from build123d import *

# Parameters (mm, degrees)
F0_R     = 2
F1_DEPTH = 1
F2_R     = 15
F3_DEPTH = 99


with BuildPart() as f1:
    # F0 (on Top) → F1 (new body)
    with BuildSketch(Plane.XY):
        with BuildLine():
            ThreePointArc((-30, -29), (-29.707107, -29.707107), (-29, -30))
            Line((-29, -30), (29, -30))
            ThreePointArc((29, -30), (29.707107, -29.707107), (30, -29))
            Line((30, -29), (30, 29))
            ThreePointArc((30, 29), (29.707107, 29.707107), (29, 30))
            Line((29, 30), (-29, 30))
            ThreePointArc((-29, 30), (-29.707107, 29.707107), (-30, 29))
            Line((-30, 29), (-30, -29))
        make_face()
        with Locations((-22.5, -22.5)):
            Circle(F0_R, mode=Mode.SUBTRACT)
        with Locations((22.5, -22.5)):
            Circle(F0_R, mode=Mode.SUBTRACT)
        with Locations((-22.5, 22.5)):
            Circle(F0_R, mode=Mode.SUBTRACT)
        with Locations((22.5, 22.5)):
            Circle(F0_R, mode=Mode.SUBTRACT)
    extrude(amount=F1_DEPTH)

    # F2 (on face) → F3 (join)
    with BuildSketch(Plane(origin=(0, 0, 0), x_dir=(1, 0, 0), z_dir=(0, 0, -1))):
        Circle(F2_R)
    extrude(amount=F3_DEPTH)


solid = f1.part
Geometry: final body of the model. Coordinates: model frame, mm. A direction names the side the tool comes from. Round coordinates to 2 decimals unless told otherwise and drop trailing zeros. Loops run counter-clockwise (first coordinate to the right, second up) from the corner with the lowest first, then second, coordinate; pieces in that order, holes last.
Q1. Section A-A on y = 22.5. Return loops of the section in (x, z).
Q2. Pin query (flat end, axial travel): P1, Ø2.5, axis at x = -22.5, y = -22.5, coming from the -Z side; P2, Ø6, axis at y = 9, z = -75, coming from the -X side; P3, Ø4, axis at y = -3, z = -24.5, coming from the -X side; P4, Ø5, axis at x = 22.5, y = -22.5, coming from the -Z side. Return the tip coordinate at first contact, or that it passes through.
Q3. Material intervals for L1, parallel to Y at x = 22.5, z = 0.75; L2, parallel to Z at x = -26.5, y = 21.5; L3, parallel to X at y = 0.5, z = -16, sorted ascending.
Q4. Pull-direction query (Y, two-part tool) for faces 1 (the cylindrical face through (-14.985, -0.66, -48.807)), 2 (the flat face through (0, 0, 1)), 3 (the cylindrical face through (-24.1, 21.3, 0.5)); classes: released by +Y, released by -Y, zero draft, split by the parting line, or undercut.
Q5. Section D-D on z = -84. Return loops of the section in (x, y).
Q6. Section C-C on x = 0. Return loops of the section in (y, z).
Q7. Access query for faces 4 (the cylindrical face through (22.24, -20.517, 0.493)), 5 (the flat face through (-7, 14, 0)). Directions: +Z, -Z, +X, -X, +Y, -Y. A direction counts if a zero-diameter tool reaches every point of the face in a straight line with its end or side. Return the directions, or none.
Evaluation:
1. outline: (-30, 0) - (-24.5, 0) - (-24.5, 1) - (-30, 1) - close; (-20.5, 0) - (20.5, 0) - (20.5, 1) - (-20.5, 1) - close; (24.5, 0) - (30, 0) - (30, 1) - (24.5, 1) - close
2. P1: passes through
2. P2: stops at x = -13.75
2. P3: stops at x = -14.97
2. P4: stops at z = 0
3. L1: y = -30 to -24.5, -20.5 to 20.5, 24.5 to 30
3. L2: z = 0 to 1
3. L3: x = -14.99 to 14.99
4. face 1: split by the parting line
4. face 2: zero draft
4. face 3: undercut
5. outline: circle Ø30 at (0, 0)
6. outline: (-30, 0) - (-15, 0) - (-15, -99) - (15, -99) - (15, 0) - (30, 0) - (30, 1) - (-30, 1) - close
7. face 4: +Z, -Z
7. face 5: -Z
